from build123d import *

# Parameters (mm, degrees)
F0_R     = 14.2875
F1_DEPTH = 12.7
F2_SIZE2 = 12.69999
F2_SIZE  = 12.69999
F3_SIZE2 = 12.69999
F3_SIZE  = 12.69999


# Not quite as in the source:
# - a fillet or chamfer is up to 0.001 mm smaller than in the source, because OpenCascade refuses the exact size


with BuildPart() as f1:
    # F0 (on Front) → F1 (new body)
    with BuildSketch(Plane.XZ):
        Polygon((-228.6, 0), (228.6, 0), (59.6845457723, 297.942), (-59.6845457723, 297.942), align=None)
        with Locations((0, 139.7)):
            Circle(F0_R, mode=Mode.SUBTRACT)
    extrude(amount=F1_DEPTH)

    # F2 (size 12.7 and 12.7 in the source; OpenCascade refuses exactly that, so slightly less here)
    f2_edges = [f1.edges().sort_by_distance(p)[0] for p in [
        (144.142273, -12.7, 148.971),
    ]]
    chamfer(f2_edges, length=F2_SIZE, length2=F2_SIZE2)

    # F3 (size 12.7 and 12.7 in the source; OpenCascade refuses exactly that, so slightly less here)
    f3_edges = [f1.edges().sort_by_distance(p)[0] for p in [
        (-144.142273, -12.7, 148.971),
    ]]
    chamfer(f3_edges, length=F3_SIZE, length2=F3_SIZE2)


solid = f1.part
Could you check a few things on this model? Use its own coordinates, in mm. Coordinates: 2 decimals unless noted, no trailing zeros. Write each loop counter-clockwise with the first axis right and the second up, starting at its lowest first coordinate (ties: lowest second). Pieces come first, ordered by that corner, then holes. Notation, with made-up numbers: (59.5, 1) - (73.5, 1) arc R18 ccw to (73.5, 29) - close; hole circle Ø5 at (-18, 57.5). An arc over 180 degrees is marked (long way). Put each result on its own line as item: value. Start each with the question number.
Q1. I want a section at A-A on x = 0. Write out the boundary of the cut face in (y, z).
Q2. Thinking about a two-plate mould opening in Z: for faces 1 (the flat face through (-3, -12.7, 118)), 2 (the cylindrical face through (-1.86, -6.261, 153.866)), 3 (the flat face through (-135.713, -6.261, 151.144)), which applies, pulls with the +Z half, pulls with the -Z half, needs draft (parallel to the pull), parting line crosses it, or undercut?
Q3. I'm going to push flat-ended pins straight in: P1, Ø6, axis at y = -2.5, z = 109, coming from the -X side; P2, Ø4, axis at y = -6.5, z = 98.5, coming from the -X side; P3, Ø5, axis at y = -11, z = 176.5, coming from the +X side. Where does each tip first touch, or does it pass through?
Q4. Please list where these lines run through material, in increasing order: L1, parallel to Z at x = 0, y = -9.25; L2, parallel to Z at x = -141, y = -12; L3, parallel to X at y = -9, z = 285.
Q5. I want a section at C-C on y = -3. Write out the boundary of the cut face in (x, z) (1 decimal), plus the area to 3 significant figures.
Checks:
1. outline: (-12.7, 0) - (0, 0) - (0, 125.41) - (-12.7, 125.41) - close; (-12.7, 153.99) - (0, 153.99) - (0, 297.94) - (-12.7, 297.94) - close
2. face 1: needs draft
2. face 2: undercut
2. face 3: pulls with the +Z half
3. P1: x = -167.74
3. P2: x = -167.85
3. P3: x = 119.09
4. L1: 0 to 125.41, 153.99 to 297.94
4. L2: 0 to 130.18
4. L3: -56.68 to 56.68
5. outline: (-225.2, 0) - (225.2, 0) - (56.2, 297.9) - (-56.2, 297.9) - close; hole circle Ø28.6 at (0, 139.7)
5. area: 83,200 mm²
